Here's how the part is built. I have some questions about the finished solid (model axes, mm). A direction names the side the tool comes from. Give positions to 0.01 mm unless a question says otherwise; leave off trailing zeros. Loops run counter-clockwise (first coordinate to the right, second up) from the corner with the lowest first, then second, coordinate; pieces in that order, holes last. Notation, with made-up numbers: (62, 62.5) - (75, 62.5) arc R34 cw to (75, 99.5) - close; hole circle Ø10 at (-3.5, 15.5). An arc over 180 degrees is marked (long way). Use a Markdown table: item, result.
from build123d import *

# Parameters (mm, degrees)
BOSS_EXTRUDE1_DEPTH = 20
SKETCH2_R           = 6.25
SKETCH2_R_2         = 4
CUT_EXTRUDE1_DEPTH  = 15
SKETCH3_R           = 9.625
SKETCH3_R_2         = 7.625
BOSS_EXTRUDE2_DEPTH = 5


with BuildPart() as part:
    # Sketch1 → Boss-Extrude1 (new body)
    with BuildSketch(Plane(origin=(0, 0, 0), x_dir=(0, 0, -1), z_dir=(1, 0, 0))):
        Polygon((0, 22), (0, 0), (23, 0), (23, -2), (0, -2), (0, -58), (-2, -58), (-2, 22), align=None)
    extrude(amount=BOSS_EXTRUDE1_DEPTH)

    # Sketch2 → Cut-Extrude1 (cut)
    with BuildSketch(Plane.XY.offset(2)):
        with Locations((10, 14)):
            Circle(SKETCH2_R)
        with Locations((10, -46)):
            Circle(SKETCH2_R_2)
    extrude(amount=-CUT_EXTRUDE1_DEPTH, mode=Mode.SUBTRACT)

    # Sketch3 → Boss-Extrude2 (add)
    with BuildSketch(Plane.XY.offset(2)):
        with Locations(Location((10, -46, 0), (0, 0, 90))):
            Circle(SKETCH3_R)
        with Locations((10, -46)):
            Circle(SKETCH3_R_2, mode=Mode.SUBTRACT)
    extrude(amount=BOSS_EXTRUDE2_DEPTH)


solid = part.part
(1) Suppose I cut it at D-D on z = 4.25. Write out the boundary of the cut face in (x, y) (3 decimals).
A:
| item | result |
|---|---|
| outline | circle Ø19.25 at (10, -46); hole circle Ø15.25 at (10, -46) |
(2) Will these pins go through, and if not, where does the flat tip stop? pin 1 (10 mm diameter, centred on x = 11.5, z = 3.5, fed in from +Y); pin 2 (12 mm diameter, centred on x = 6.5, y = 11.5, fed in from -Z); pin 3 (3 mm diameter, centred on x = 7, z = -5, fed in from -Y); pin 4 (1.5 mm diameter, centred on x = 6, y = -30.5, fed in from +Z).
A:
| item | result |
|---|---|
| pin 1 | y = 22 |
| pin 2 | z = 0 |
| pin 3 | y = -2 |
| pin 4 | z = 2 |
(3) If I drill on line 1 (Y direction, x = 10, z = 1.3); line 2 (Y direction, x = 6.25, z = -21.5); line 3 (Z direction, x = 18, y = -35.5), over which ranges is the centre line in solid material (lowest first)?
A:
| item | result |
|---|---|
| line 1 | -58 to -50, -42 to 7.75, 20.25 to 22 |
| line 2 | -2 to 0 |
| line 3 | 0 to 2 |
(4) We'd pull the mould along Y, two halves only. Please class faces 5 (the face through (17.044, -48.92, 4.465)), 6 (the face through (15.857, -53.638, 4.465)), 7 (the face through (10, -2, -12)), 8 (the face through (10, 6, 0)): pulls with the +Y half, pulls with the -Y half, needs draft (parallel to the pull), parting line crosses it, or undercut.
A:
| item | result |
|---|---|
| face 5 | undercut |
| face 6 | parting line crosses it |
| face 7 | pulls with the -Y half |
| face 8 | needs draft |
(5) Suppose I cut it at B-B on y = 14. Write out the boundary of the cut face in (x, z).
A:
| item | result |
|---|---|
| outline | (0, 0) - (3.75, 0) - (3.75, 2) - (0, 2) - close; (16.25, 0) - (20, 0) - (20, 2) - (16.25, 2) - close |
(6) Suppose I cut it at C-C on x = 18.5. Write out the boundary of the cut face in (y, z).
A:
| item | result |
|---|---|
| outline | (-58, 0) - (-2, 0) - (-2, -23) - (0, -23) - (0, 0) - (22, 0) - (22, 2) - (-41.48, 2) - (-41.48, 7) - (-50.52, 7) - (-50.52, 2) - (-58, 2) - close |
(7) Suppose I cut it at A-A on x = 10. Write out the boundary of the cut face in (y, z) (3 decimals).
A:
| item | result |
|---|---|
| outline | (-58, 0) - (-50, 0) - (-50, 2) - (-53.625, 2) - (-53.625, 7) - (-55.625, 7) - (-55.625, 2) - (-58, 2) - close; (-42, 0) - (-2, 0) - (-2, -23) - (0, -23) - (0, 0) - (7.75, 0) - (7.75, 2) - (-36.375, 2) - (-36.375, 7) - (-38.375, 7) - (-38.375, 2) - (-42, 2) - close; (20.25, 0) - (22, 0) - (22, 2) - (20.25, 2) - close |
(8) On a 3-axis mill with a long thin cutter (end or side, diameter ignored), from which of +Z, -Z, +X, -X, +Y, -Y can I reach the whole of each face in a straight line? I mean faces 1 (the face through (10, 0, -11)), 2 (the face through (13, -43, 2)), 3 (the face through (7.05, -43.3, 1.01)), 4 (the face through (10, -30, 0)). Say none if no direction works.
A:
| item | result |
|---|---|
| face 1 | -Z, +X, -X, +Y |
| face 2 | +Z |
| face 3 | +Z, -Z |
| face 4 | -Z, +X, -X, -Y |
